Could you check a few things on this model? Use its own coordinates, in mm. A direction names the side the tool comes from. Give positions to 0.01 mm unless a question says otherwise; leave off trailing zeros. Loops run counter-clockwise (first coordinate to the right, second up) from the corner with the lowest first, then second, coordinate; pieces in that order, holes last. Notation, with made-up numbers: (53, 21) - (77, 21) arc R27 ccw to (77, 56) - close; hole circle Ø6 at (46, 15.5). An arc over 180 degrees is marked (long way). Use CSV: the item, a comma, the result in double quotes.
Autodesk Inventor part; units mm, degrees
ref_plane "YZ Plane" through (0, 0, 0) normal (1, 0, 0) x (0, 1, 0)
ref_plane "XZ Plane" through (0, 0, 0) normal (0, 1, 0) x (-1, 0, 0)
ref_plane "XY Plane" through (0, 0, 0) normal (0, 0, 1) x (1, 0, 0)
sketch "Sketch1" plane through (0, 0, 0) normal (0, 1, 0) x (-1, 0, 0)
  line L0 (-6.35, 6.35) -> (6.35, 6.35)
  line L1 (6.35, 6.35) -> (6.35, -6.35)
  line L2 (6.35, -6.35) -> (-6.35, -6.35)
  line L3 (-6.35, -6.35) -> (-6.35, 6.35)
  line L4 (-6.35, 6.35) -> (6.35, -6.35) construction
  line L5 (6.35, 6.35) -> (-6.35, -6.35) construction
  circle A0 centre (0, 0) radius 4.7625
  dimension "d0" = 12.7
  dimension "d1" = 12.7
  dimension "d2" = 9.525
extrude "Extrusion1" add sketch "Sketch1" along normal blind 12.7
sketch "Sketch2" plane through (-6.35, 0, 6.35) normal (0, 0, 1) x (1, 0, 0)
  line L0 (6.35, 0) -> (6.35, 6.35)
  circle A0 centre (6.35, 6.35) radius 1.5875
  dimension "d5" = 6.35
  dimension "d6" = 3.175
extrude "Extrusion2" add sketch "Sketch2" against normal blind 4.445
sketch "Sketch3" plane through (-6.35, 0, 6.35) normal (0, 0, 1) x (1, 0, 0)
  line L0 (12.7, 0) -> (0, 0)
  line L1 (12.7, 0) -> (12.7, 12.7)
  line L2 (0, 0) -> (12.7, 0)
  line L3 (12.7, 0) -> (12.7, 12.7)
  line L4 (12.7, 12.7) -> (0, 12.7)
  line L5 (0, 12.7) -> (0, 0)
  point P0 (6.35, 0)
extrude "Extrusion3" add sketch "Sketch3" along normal blind 127
fillet "Fillet1" radius 2.54 12 edges at (6.35, 12.7, 63.5) (6.35, 0, 63.5) (-6.35, 12.7, 63.5) (-6.35, 0, 63.5) (-6.35, 6.35, 133.35) (0, 0, 133.35) (6.35, 6.35, 133.35) (0, 12.7, 133.35) (-6.35, 6.35, -6.35) (6.35, 6.35, -6.35) (0, 12.7, -6.35) (0, 0, -6.35)
sketch "Sketch4" plane through (0, 12.7, 0) normal (0, 1, 0) x (1, 0, 0)
  line L0 (0, 0) -> (0, -101.854)
  line L1 (0, 0) -> (101.854, 0) construction
  dimension "d12" = 101.854
  dimension "d13" = 90
hole "Hole1" at (0, 12.7, 101.854) direction (0, -1, 0) diameter 5.4102 depth 6.35
hole "Hole2" at (0, 12.7, 101.854) direction (0, -1, 0) diameter 3.175 depth 25.4 tip angle 118
sketch "Sketch5" plane through (-6.35, 2.54, -3.81) normal (-1, 0, 0) x (0, 0, 1)
  line L0 (3.81, -2.54) -> (96.774, -2.54)
  line L1 (3.81, -2.54) -> (96.774, -2.54) construction
  line L2 (96.774, -2.54) -> (96.774, 3.81)
  line L3 (134.62, 0) -> (0, 0)
  line L4 (96.774, -2.54) -> (103.124, -2.54) construction
  point P0 (3.81, 10.16)
  dimension "d28" = 92.964
  dimension "d29" = 0
  dimension "d30" = 6.35
  dimension "d31" = 90
hole "Hole3" at (-6.35, 6.35, 92.964) direction (1, 0, 0) diameter 5.4102 depth 6.35
properties part number "spincoater dispense arm"
1) I need wall thicknesses on line 1 along Z through (x, y) = (2.25, 11.25); line 2 along Z through (x, y) = (-2.25, 7.5); line 3 along Y through (x, z) = (-4, 28). Which ranges of each line are inside material? Lowest first, please.
Answer below:
line 1,"z = -6.1 to -4.2, 4.2 to 100.35, 103.36 to 133.1"
line 2,"z = -6.35 to -4.2, 4.2 to 90.52, 95.41 to 100.35, 103.36 to 133.35"
line 3,"y = 0.01 to 12.69"
2) Suppose I cut it at A-A (z = 46). Please give me the cut outline in (x, y), plus the area to 3 significant figures.
Answer below:
outline,"(-6.35, 2.54) arc R2.54 ccw to (-3.81, 0) - (3.81, 0) arc R2.54 ccw to (6.35, 2.54) - (6.35, 10.16) arc R2.54 ccw to (3.81, 12.7) - (-3.81, 12.7) arc R2.54 ccw to (-6.35, 10.16) - close"
area,"156 mm2"
3) I'm going to push a flat-ended pin straight in: P1, Ø5, axis at x = 0, z = 101.854, coming from the +Y side. Where does the tip first touch, or does it pass through?
Answer below:
P1,"stops at y = 6.35"
4) We'd pull the mould along Y, two halves only. Please class faces 5 (the cylindrical face through (-5.626, 6.403, 132.586)), 6 (the flat face through (0, 0, 66)), 7 (the cylindrical face through (-3.13, 7.39, 95.46)), 8 (the cylindrical face through (0.053, 11.976, 132.586)): +Y half, -Y half, draft (parallel to the pull), parting line (faces both ways), or undercut.
Answer below:
face 5,"draft"
face 6,"-Y half"
face 7,"undercut"
face 8,"+Y half"
5) Which directions (+Z, -Z, +X, -X, +Y, -Y) give clear straight access to the entire face, cutting with the end or side of a thin tool? Please do faces 1 (the flat face through (0, 6, 1.905)), 2 (the cylindrical face through (5.626, 6.297, 132.586)), 3 (the cylindrical face through (1.466, 5.742, 3.354)), 4 (the cylindrical face through (1.04, 9.48, 104.35)).
Answer below:
face 1,"+Y, -Y"
face 2,"+Z, +X, +Y, -Y"
face 3,"none"
face 4,"+Y"
6) Suppose I cut it at B-B (z = 0). Please give me the cut outline in (x, y).
Answer below:
outline,"(-6.35, 2.54) arc R2.54 ccw to (-4.76, 0.19) - (-4.76, 12.51) arc R2.54 ccw to (-6.35, 10.16) - close; (4.76, 0.19) arc R2.54 ccw to (6.35, 2.54) - (6.35, 10.16) arc R2.54 ccw to (4.76, 12.51) - close"
